Design review of the part shown in the three views and the two pictorial views. Dimensions are in mm from the part's minimum x, y and z. Give positions to 0.01 mm unless a question says otherwise; leave off trailing zeros. Loops run counter-clockwise (first coordinate to the right, second up) from the corner with the lowest first, then second, coordinate; pieces in that order, holes last. Notation, with made-up numbers: (64, 21.5) - (120, 21.5) arc R14 ccw to (120, 33.5) - close; hole circle Ø3 at (89.25, 74). An arc over 180 degrees is marked (long way). Use CSV: the item, a comma, the result in double quotes. Start each with the question number.
1. Take a section at D-D on x = 7.5. Give the boundary of the cut face in (y, z) (1 decimal), plus the area to 3 significant figures.
2. For pin 1 (5 mm diameter, centred on x = 5, y = 7, fed in from +Z); pin 2 (2 mm diameter, centred on y = 4.5, z = 23, fed in from -X); pin 3 (5 mm diameter, centred on x = 3.5, z = 21, fed in from -Y); pin 4 (1 mm diameter, centred on x = 21.5, y = 2, fed in from +Z), all flat-tipped, find the tip position at first contact; note any pin that passes through.
3. Take a section at B-B on z = 16. Give the boundary of the cut face in (x, y), plus the area to 3 significant figures.
4. Wall thickness on line 1 (Z direction, x = 16, y = 13); line 2 (Z direction, x = 16, y = 4.25); line 3 (Y direction, x = 28, z = 26.5): over which ranges is each line inside the solid? List them lowest first.
5. Mouldability with a two-part tool opening along X and no side actions: class the marked faces 1, 2 and 3 as pulls with the +X half, pulls with the -X half, needs draft (parallel to the pull), parting line crosses it, or undercut.
6. Take a section at C-C on y = 11.25. Give the boundary of the cut face in (x, z).
7. Take a section at A-A on x = 16. Give the boundary of the cut face in (y, z), plus the area to 3 significant figures.
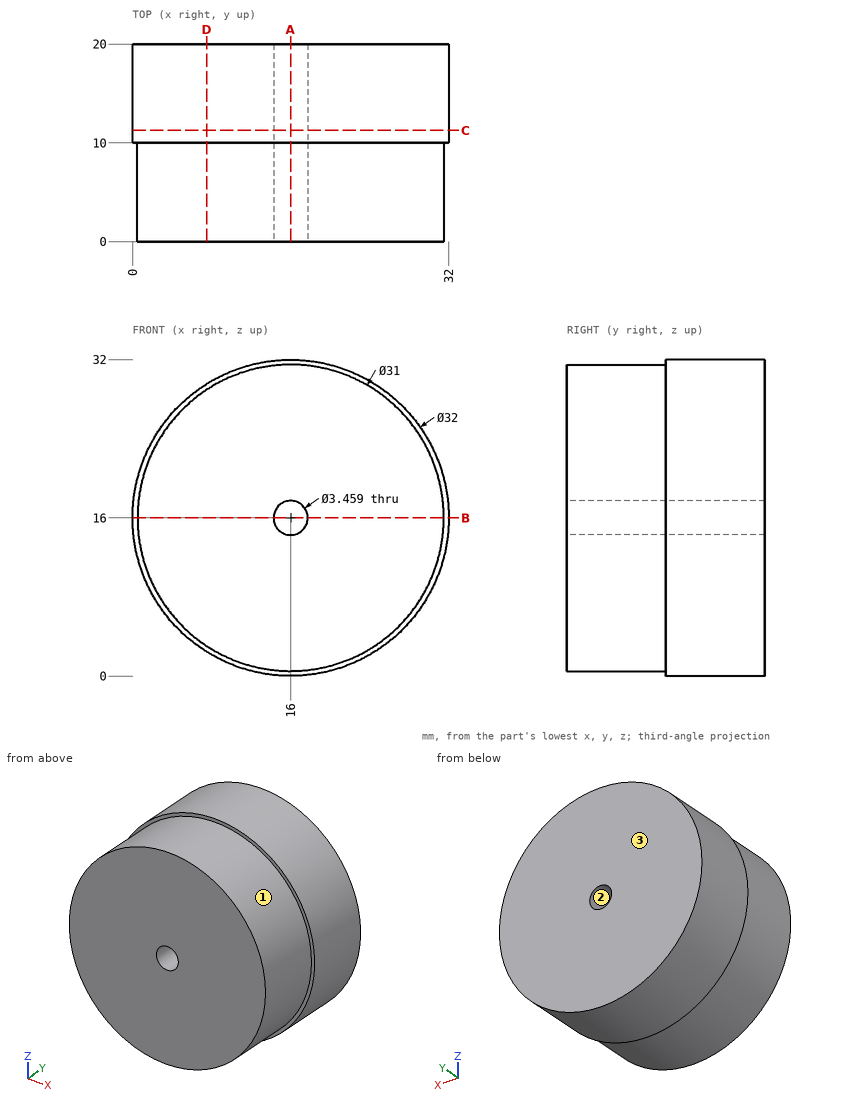
Check result:
1,outline,"(0, 3) - (10, 3) - (10, 2.4) - (20, 2.4) - (20, 29.6) - (10, 29.6) - (10, 29) - (0, 29) - close"
1,area,"530 mm²"
2,pin 1,"stops at z = 28.96"
2,pin 2,"stops at x = 1.71"
2,pin 3,"stops at y = 0"
2,pin 4,"stops at z = 30.67"
3,outline,"(0, 10) - (0.5, 10) - (0.5, 0) - (14.27, 0) - (14.27, 20) - (0, 20) - close; (17.73, 0) - (31.5, 0) - (31.5, 10) - (32, 10) - (32, 20) - (17.73, 20) - close"
3,area,"561 mm²"
4,line 1,"z = 0 to 14.27, 17.73 to 32"
4,line 2,"z = 0.5 to 14.27, 17.73 to 31.5"
4,line 3,"y = 10 to 20"
5,face 1,"parting line crosses it"
5,face 2,"undercut"
5,face 3,"needs draft"
6,outline,"circle Ø32 at (16, 16); hole circle Ø3.46 at (16, 16)"
7,outline,"(0, 0.5) - (10, 0.5) - (10, 0) - (20, 0) - (20, 14.27) - (0, 14.27) - close; (0, 17.73) - (20, 17.73) - (20, 32) - (10, 32) - (10, 31.5) - (0, 31.5) - close"
7,area,"561 mm²"
